Autodesk Inventor part; units mm, degrees
ref_plane "YZ Plane" through (0, 0, 0) normal (1, 0, 0) x (0, 1, 0)
ref_plane "XZ Plane" through (0, 0, 0) normal (0, 1, 0) x (-1, 0, 0)
ref_plane "XY Plane" through (0, 0, 0) normal (0, 0, 1) x (1, 0, 0)
sketch "Skizze1" plane through (0, 0, 0) normal (1, 0, 0) x (0, 1, 0)
  line L0 (5, 22) -> (-5, 22)
  line L1 (-5, 22) -> (-5, 20)
  line L2 (-5, 20) -> (5, 20)
  line L3 (5, 20) -> (5, 22)
  line L4 (5.4713, 0) -> (-6.5925, 0)
  point P0 (0, 0)
  point P1 (0, 20)
  point P2 (0, 22)
  dimension "d0" = 20
  dimension "d1" = 22
  dimension "d2" = 10
  dimension "d3" = 5
revolve "Basebody" add sketch "Skizze1" angle 360 about axis through (0, 5.4713, 0) along (0, -1, 0)
chamfer "Fasen1" distance 0.5 angle 45 4 edges at (0, 5, -20) (0, 5, -22) (0, -5, -22) (0, -5, -20)
properties part number "35-30-xxx Plain Bearing Socket" material "Kunststoff, undurchsichtig Weiß"
Verification items for the finished model (mm, model axes). Round coordinates to 2 decimals unless told otherwise and drop trailing zeros. Write each loop counter-clockwise with the first axis right and the second up, starting at its lowest first coordinate (ties: lowest second). Pieces come first, ordered by that corner, then holes. Notation, with made-up numbers: (55.5, -28.75) -> (63.5, -28.75) arc R22 cw to (63.5, -20.75) -> close; hole circle Ø1 at (-39, 29). An arc over 180 degrees is marked (long way). Write each question's results on one line, items separated by ' | '.
Q1. Sectioned sample at A-A, the plane z = 0. Record the boundary of the cut face in (x, y), and give its area (3 significant figures).
Derived:
outline: (-22, -4.5) -> (-21.5, -5) -> (-20.5, -5) -> (-20, -4.5) -> (-20, 4.5) -> (-20.5, 5) -> (-21.5, 5) -> (-22, 4.5) -> close; (20, -4.5) -> (20.5, -5) -> (21.5, -5) -> (22, -4.5) -> (22, 4.5) -> (21.5, 5) -> (20.5, 5) -> (20, 4.5) -> close | area: 39.0 mm²
Q2. Sectioned sample at B-B, the plane x = 0. Record the boundary of the cut face in (y, z).
Derived:
outline: (-5, -21.5) -> (-4.5, -22) -> (4.5, -22) -> (5, -21.5) -> (5, -20.5) -> (4.5, -20) -> (-4.5, -20) -> (-5, -20.5) -> close; (-5, 20.5) -> (-4.5, 20) -> (4.5, 20) -> (5, 20.5) -> (5, 21.5) -> (4.5, 22) -> (-4.5, 22) -> (-5, 21.5) -> close
Q3. Thickness scan on probe 1 along X at (y, z) = (-0.5, 0); probe 2 along X at (y, z) = (0.75, -5). Record the ranges inside material, lowest first.
Derived:
probe 1: x = -22 to -20, 20 to 22 | probe 2: x = -21.42 to -19.36, 19.36 to 21.42
Q4. Draft check along Z on faces 1 (the face through (21.477, -0.063, -4.769)), 2 (the face through (21, 5, 0)), 3 (the face through (-19.524, 0.063, -4.336)). Enter one of: released by +Z, released by -Z, zero draft, split by the parting line, or undercut.
Derived:
face 1: split by the parting line | face 2: zero draft | face 3: undercut
Q5. Go/stop test with flat-tipped pins: pin 1 Ø2 at (y, z) = (-0.5, -6.5) entering from +X; pin 2 Ø2 at (y, z) = (0, -16.5) entering from +X; pin 3 Ø6 at (y, z) = (-1, -12.5) entering from -X. Record where each tip stops, or that it passes through.
Derived:
pin 1: stops at x = 21.3 | pin 2: stops at x = 15.61 | pin 3: stops at x = -19.84
Q6. Sectioned sample at C-C, the plane y = -2.5. Record the boundary of the cut face in (x, z).
Derived:
outline: circle Ø44 at (0, 0); hole circle Ø40 at (0, 0)
